Model file for the job. Use its own axes, mm. A direction names the side the tool comes from. Give positions to 0.01 mm unless a question says otherwise; leave off trailing zeros. Order: outer loops, then holes, each group sorted by start corner. A loop starts at its lowest first (then second) coordinate and runs counter-clockwise, first axis right, second up. Notation, with made-up numbers: (65, -7.5) - (117, -7.5) arc R11 cw to (117, 7.5) - close; hole circle Ø7 at (62, -18). An arc over 180 degrees is marked (long way). Use CSV: the item, a comma, the result in double quotes. Start each with the question number.
(1) Band-saw the part on C-C, the plane x = 15. Give the cut face in (y, z).
(2) Band-saw the part on A-A, the plane z = 10.75. Count the separate pieces of the cut face and the enclosed holes in it, then the cut area to 3 significant figures.
(3) Tool access for faces 5 (the flat face through (22, 1, 10)), 6 (the flat face through (14.2, 0.7, 0)): list every direction of +Z, -Z, +X, -X, +Y, -Y with a clear straight run to the whole face (end or side of a thin tool).
(4) Pull direction X, two halves, no side cores. Call faces 1 (the flat face through (0.5, 20, 9.9)), 2 (the cylindrical face through (16.56, 0.51, 11.45)), 3 (the flat face through (0, 5, 8)), 4 (the flat face through (40, 0.5, 9.9)): +X half, -X half, draft (parallel to the pull), parting line (faces both ways), or undercut.
(5) Probe L1, parallel to Y at x = 11.5, z = 3; L2, parallel to X at y = 2.75, z = 2.25. List the from-to ranges inside material, lowest first.
(6) Drop flat-ended pins along their axis: pin 1 Ø1 at (y, z) = (5, 4.5) entering from +X; pin 2 Ø10 at (x, z) = (15, 9) entering from +Y; pin 3 Ø11 at (x, y) = (5, 5.5) entering from +Z. Give the stop position or say it passes through.
(7) Band-saw the part on B-B, the plane y = 8.25. Give the cut face in (x, z).
from build123d import *

# Parameters (mm, degrees)
EXTRUDE1_DEPTH     = 20
FILLET1_R          = 2.54
SKETCH8_R          = 5.014710823
CUT_EXTRUDE2_DEPTH = 10
CUT_EXTRUDE5_DEPTH = 10
SKETCH10_R         = 1.5
CUT_EXTRUDE6_DEPTH = 10
SKETCH11_R         = 1.5
CUT_EXTRUDE7_DEPTH = 30


with BuildPart() as part:
    # Sketch1 → Extrude1 (new body)
    with BuildSketch(Plane.XY):
        Polygon((1, 20), (1, 1), (40, 1), (40, 0), (0, 0), (0, 20), align=None)
    extrude(amount=EXTRUDE1_DEPTH)

    # Fillet1
    fillet1_edges = [part.edges().sort_by_distance(p)[0] for p in [
        (1, 1, 10),
    ]]
    fillet(fillet1_edges, radius=FILLET1_R)

    # Sketch8 → Cut-Extrude2 (cut)
    with BuildSketch(Plane.ZY):
        with Locations((10.002916517, 10.036253446)):
            Circle(SKETCH8_R)
    extrude(amount=-CUT_EXTRUDE2_DEPTH, mode=Mode.SUBTRACT)

    # Sketch9 → Cut-Extrude5 (cut)
    with BuildSketch(Plane.ZY):
        with BuildLine():
            Line((20, 20), (11.343762255, 20))
            ThreePointArc((11.343762255, 20), (17.466219012, 17.238892052), (19.972229781, 11.007671958))
            Line((19.972229781, 11.007671958), (19.972229781, 0.025510204))
            Line((19.972229781, 0.025510204), (0, 0.025510204))
            Line((0, 0.025510204), (0, 0))
            Line((0, 0), (20, 0))
            Line((20, 0), (20, 12.992821057))
            Line((20, 12.992821057), (20, 20))
        make_face()
        with BuildLine():
            ThreePointArc((8.27076822, 19.981825104), (8.425722381, 19.992250227), (8.580833361, 20))
            Line((8.580833361, 20), (0, 20))
            Line((0, 20), (0, 11.932412977))
            ThreePointArc((0, 11.932412977), (2.62467317, 17.407695827), (8.129433274, 19.969969766))
            ThreePointArc((8.129433274, 19.969969766), (8.200077393, 19.976175852), (8.27076822, 19.981825104))
        make_face()
    extrude(amount=-CUT_EXTRUDE5_DEPTH, mode=Mode.SUBTRACT)

    # Sketch10 → Cut-Extrude6 (cut)
    with BuildSketch(Plane(origin=(0, 1, 0), x_dir=(1, 0, 0), z_dir=(0, 1, 0))):
        with Locations((15.871397646, -10.116419243)):
            Circle(SKETCH10_R)
    extrude(amount=-CUT_EXTRUDE6_DEPTH, mode=Mode.SUBTRACT)

    # Sketch11 → Cut-Extrude7 (cut)
    with BuildSketch(Plane(origin=(0, 1, 0), x_dir=(1, 0, 0), z_dir=(0, 1, 0))):
        with Locations((34.079367283, -10.116419243)):
            Circle(SKETCH11_R)
    extrude(amount=-CUT_EXTRUDE7_DEPTH, mode=Mode.SUBTRACT)


solid = part.part
Answer block:
1,outline,"(0, 0) - (1, 0) - (1, 8.9) - (0, 8.9) - close; (0, 11.34) - (1, 11.34) - (1, 20) - (0, 20) - close"
2,separate pieces,"4"
2,enclosed holes,"0"
2,area,"44.8 mm2"
3,face 5,"+Z, -Z, +X, +Y"
3,face 6,"-Z, +X, -X, +Y, -Y"
4,face 1,"draft"
4,face 2,"undercut"
4,face 3,"-X half"
4,face 4,"+X half"
5,L1,"y = 0 to 1"
5,L2,"x = 0 to 1.13"
6,pin 1,"stops at x = 1"
6,pin 2,"stops at y = 1"
6,pin 3,"stops at z = 19.97"
7,outline,"(0, 0) - (1, 0) - (1, 5.32) - (0, 5.32) - close; (0, 14.69) - (1, 14.69) - (1, 19.97) - (0, 19.97) - close"
